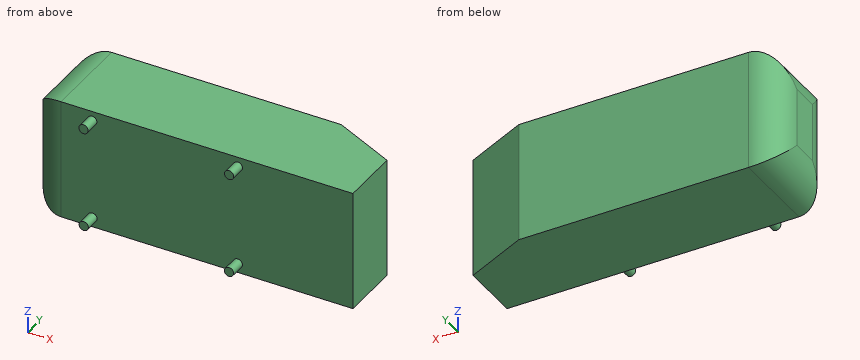
```python
from build123d import *

# Parameters (mm, degrees)
F1_DEPTH = 389
F2_R     = 100
F7_R     = 15
F8_DEPTH = 50
F5_R     = 15
F4_R     = 15
F6_R     = 15
F9_DEPTH = 50


with BuildPart() as f1:
    # F0 (on Top) → F1 (new body)
    with BuildSketch(Plane.XY):
        Polygon((-1044, 288.001959), (-1044, 0), (0, 0), (0, 194.18), (-201.2, 288.001959), align=None)
    extrude(amount=-F1_DEPTH)

    # F2
    f2_edges = [f1.edges().sort_by_distance(p)[0] for p in [
        (-1044, 288.001959, -194.5),
        (-1044, 0, -194.5),
        (-1044, 144.00098, 0),
        (-1044, 144.00098, -389),
    ]]
    fillet(f2_edges, radius=F2_R)

    # F7 (on offset) → F8 (join)
    with BuildSketch(Plane.XZ.offset(50)):
        with Locations((-842.109799, -357.525885)):
            Circle(F7_R)
    extrude(amount=-F8_DEPTH)

    # F5 (on offset) + F4 (on offset) + F6 (on offset) → F9 (join)
    with BuildSketch(Plane.XZ.offset(50)):
        with Locations((-372.279406, -358.30304)):
            Circle(F5_R)
    with BuildSketch(Plane.XZ.offset(50)):
        with Locations((-372, -31)):
            Circle(F4_R)
    with BuildSketch(Plane.XZ.offset(50)):
        with Locations((-843.018532, -30.759659)):
            Circle(F6_R)
    extrude(amount=-F9_DEPTH)


solid = f1.part
```
Input: part model. Units: mm. Frame: model coordinates. Give positions to 0.01 mm unless a question says otherwise; leave off trailing zeros. Order: outer loops, then holes, each group sorted by start corner. A loop starts at its lowest first (then second) coordinate and runs counter-clockwise, first axis right, second up. Notation, with made-up numbers: M -28.5,3 L -16.5,3 A18 ccw -16.5,37 Z; hole C -13,-28 d11. An arc over 180 degrees is marked long. Return JSON: item names as keys, results as strings.
Item 1: Cut plane D-D (z = -315). Return loops of the section in (x, y), then the cut area to 3 significant figures.
Solutions:
{"outline": "M -1040.56,74 A100 ccw -944,0 L 0,0 L 0,194.18 L -201.2,288 L -944,288 A100 ccw -1040.56,214 Z", "area": "287,000 mm^2"}
Item 2: Cut plane C-C (y = 261). Return loops of the section in (x, z).
Solutions:
{"outline": "M -1012.35,-362 A100 ccw -944,-389 L -143.29,-389 L -143.29,0 L -944,0 A100 ccw -1012.35,-27 Z"}
Item 3: Ray query, probe 1 along Y at (x, z) = (-534.5, -249.5); probe 2 along X at (y, z) = (78, -78.5); probe 3 along X at (y, z) = (31, -176). Return the intervals inside material, ascending.
Solutions:
{"probe 1": "0 to 288", "probe 2": "-1041.55 to 0", "probe 3": "-1016.38 to 0"}
Item 4: Cut plane B-B (x = -266.5). Return loops of the section in (y, z), then the cut area to 3 significant figures.
Solutions:
{"outline": "M 0,-389 L 288,-389 L 288,0 L 0,0 Z", "area": "112,000 mm^2"}
Item 5: First-contact query: P1, Ø5, axis at y = 100.5, z = -324.5, coming from the -X side; P2, Ø4, axis at y = 16, z = -227.5, coming from the -X side; P3, Ø4, axis at x = -224, z = -198, coming from the -Y side. Flat tips, straight axial feed; report the tip coordinate or a pass-through.
Solutions:
{"P1": "x = -1038.4", "P2": "x = -1001.24", "P3": "y = 0"}
Item 6: Cut plane A-A (z = -191). Return loops of the section in (x, y).
Solutions:
{"outline": "M -1044,100 A100 ccw -944,0 L 0,0 L 0,194.18 L -201.2,288 L -944,288 A100 ccw -1044,188 Z"}
